Check sheet for the modelled part. Datum: model origin and axes. Units: mm. A direction names the side the tool comes from. Round coordinates to 2 decimals unless told otherwise and drop trailing zeros. Loops run counter-clockwise (first coordinate to the right, second up) from the corner with the lowest first, then second, coordinate; pieces in that order, holes last. Notation, with made-up numbers: (22.5, -33.75) -> (74.5, -33.75) arc R29 ccw to (74.5, -9.75) -> close; hole circle Ø1 at (53, 29.5). An arc over 180 degrees is marked (long way). Return JSON: item names as keys, results as strings.
from build123d import *

# Parameters (mm, degrees)
F0_R      = 10.0048982814
F0_R_2    = 8.7765216672
F1_DEPTH  = 1.99898
F0_R_3    = 3.608871
F2_DEPTH  = 5.9944
F3_DEPTH  = 10.1092
F4_R      = 3.7405824935
F5_R      = 4.7625
F6_DEPTH  = 1.016
F7_R      = 0.2452840979
F8_R      = 3.608871
F8_R_2    = 3.3131091119
F9_DEPTH  = 2.7686
F8_R_3    = 2.6420381333
F10_DEPTH = 2.032
F13_DEPTH = 0.127
F14_DEPTH = 0.508
F15_DEPTH = 0.05334


with BuildPart() as f1:
    # F0 (on Top) → F1 (new body)
    with BuildSketch(Plane.XY):
        Circle(F0_R)
        Circle(F0_R_2, mode=Mode.SUBTRACT)
    extrude(amount=F1_DEPTH)

    # F0 (on Top) → F2 (join)
    with BuildSketch(Plane.XY):
        Circle(F0_R_2)
        Circle(F0_R_3, mode=Mode.SUBTRACT)
        Circle(F0_R_3)
    extrude(amount=F2_DEPTH)

    # F0 (on Top) → F3 (join)
    with BuildSketch(Plane.XY):
        Circle(F0_R_3)
    extrude(amount=F3_DEPTH)

    # F4
    f4_edges = [f1.edges().sort_by_distance(p)[0] for p in [
        (-8.776522, 0, 5.9944),
    ]]
    fillet(f4_edges, radius=F4_R)

    # F5 (on face) → F6 (join)
    with BuildSketch(Plane.XY.offset(5.9944)):
        Circle(F5_R)
    extrude(amount=F6_DEPTH)

    # F7
    f7_edges = [f1.edges().sort_by_distance(p)[0] for p in [
        (-4.7625, 0, 7.0104),
    ]]
    fillet(f7_edges, radius=F7_R)

    # F8 (on face) → F9 (cut)
    with BuildSketch(Plane.XY.offset(10.1092)):
        Circle(F8_R)
        Circle(F8_R_2, mode=Mode.SUBTRACT)
    extrude(amount=-F9_DEPTH, mode=Mode.SUBTRACT)

    # F8 (on face) → F10 (cut)
    with BuildSketch(Plane.XY.offset(10.1092)):
        Circle(F8_R_2)
        Circle(F8_R_3, mode=Mode.SUBTRACT)
    extrude(amount=-F10_DEPTH, mode=Mode.SUBTRACT)

    # F12 (on offset) → F13 (join, symmetric)
    with BuildSketch(Plane.XZ.offset(-2.667)):
        with BuildLine():
            ThreePointArc((0.6982848187, 9.1637990087), (0.4936989053, 9.6577130953), (-0.0002151813, 9.8622990087))
            Line((-0.0002151813, 9.8622990087), (-0.0002151813, 9.3522478652))
            ThreePointArc((-0.0002151813, 9.3522478652), (0.1330382831, 9.2970524731), (0.1882336753, 9.1637990087))
            ThreePointArc((0.1882336753, 9.1637990087), (0.1330382831, 9.0305455443), (-0.0002151813, 8.9753501521))
            Line((-0.0002151813, 8.9753501521), (-0.0002151813, 8.4652990087))
            ThreePointArc((-0.0002151813, 8.4652990087), (0.4936989053, 8.669884922), (0.6982848187, 9.1637990087))
        make_face()
        with BuildLine():
            Line((-0.0002151813, 9.3522478652), (-0.0002151813, 9.8622990087))
            ThreePointArc((-0.0002151813, 9.8622990087), (-0.6987151813, 9.1637990087), (-0.0002151813, 8.4652990087))
            Line((-0.0002151813, 8.4652990087), (-0.0002151813, 8.9753501521))
            ThreePointArc((-0.0002151813, 8.9753501521), (-0.1886640379, 9.1637990087), (-0.0002151813, 9.3522478652))
        make_face()
    extrude(amount=F13_DEPTH, both=True)

    # F12 (on offset) → F14 (cut)
    with BuildSketch(Plane.XZ.offset(-2.667)):
        with BuildLine():
            ThreePointArc((0.1882336753, 9.1637990087), (0.1330382831, 9.2970524731), (-0.0002151813, 9.3522478652))
            Line((-0.0002151813, 9.3522478652), (-0.0002151813, 8.9753501521))
            ThreePointArc((-0.0002151813, 8.9753501521), (0.1330382831, 9.0305455443), (0.1882336753, 9.1637990087))
        make_face()
        with BuildLine():
            Line((-0.0002151813, 8.9753501521), (-0.0002151813, 9.3522478652))
            ThreePointArc((-0.0002151813, 9.3522478652), (-0.1886640379, 9.1637990087), (-0.0002151813, 8.9753501521))
        make_face()
    extrude(amount=F14_DEPTH, mode=Mode.SUBTRACT)

    # F8 (on face) → F15 (cut)
    with BuildSketch(Plane.XY.offset(10.1092)):
        Polygon((0.008962602, 1.624630818), (-1.0713262968, -0.2752078575), (-0.6395262968, -0.2772395093), (0.0069309502, 1.192830818), (0.5111417182, -0.2826534897), (0.9429417182, -0.2846851415), align=None)
    extrude(amount=-F15_DEPTH, mode=Mode.SUBTRACT)


solid = f1.part
Q1. Section check B-B (z = 2.5). Record the boundary of the cut face in (x, y).
Results list:
{"outline": "circle Ø17.54 at (0, 0)"}
Q2. Material ranges on line 1 (Z direction, x = 2, y = -3.75); line 2 (Z direction, x = -0.5, y = -3); line 3 (Y direction, x = 0, z = 7.75), recorded low to high.
Results list:
{"line 1": "0 to 7.01", "line 2": "0 to 8.08", "line 3": "-3.31 to 3.31"}
Q3. Section check A-A (z = 5.25). Record the boundary of the cut face in (x, y).
Results list:
{"outline": "circle Ø14.55 at (0, 0)"}
Q4. Tool access check on faces 1 (the flat face through (0, 0, 10.109)), 2 (the cylindrical face through (3.334, -1.382, 7.173)). Record the directions out of +Z, -Z, +X, -X, +Y, -Y that give a thin tool (end or side, any length) a straight path to the whole face; none if there is none.
Results list:
{"face 1": "+Z, +X, -X, +Y, -Y", "face 2": "+Z"}
Q5. Go/stop test with flat-tipped pins: pin 1 (1.5 mm diameter, centred on y = -3, z = 4, fed in from -X); pin 2 (0.7 mm diameter, centred on x = 0, z = 9.5, fed in from +Y); pin 3 (2 mm diameter, centred on x = 6.5, z = 8, fed in from +Y); pin 4 (1 mm diameter, centred on x = -4, y = 8, fed in from +Z) (3 decimals). Record where each tip stops, or that it passes through.
Results list:
{"pin 1": "x = -8.21", "pin 2": "y = 2.79", "pin 3": "through", "pin 4": "z = 3.795"}
Q6. Draft check along Y on faces 3 (the flat face through (0, 0, 0)), 4 (the cylindrical face through (-0.57, -2.58, 9.11)). Enter one of: released by +Y, released by -Y, zero draft, split by the parting line, or undercut.
Results list:
{"face 3": "zero draft", "face 4": "split by the parting line"}
